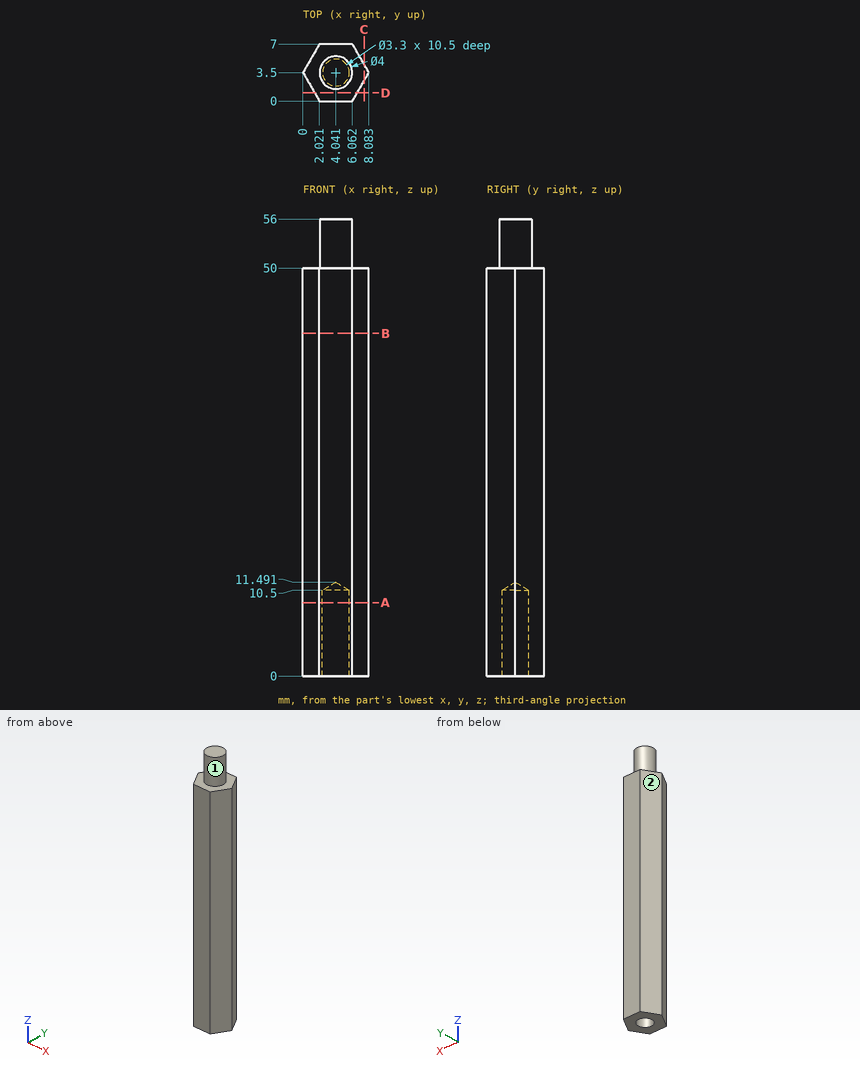
The figure shows three views and two pictorial views of one solid part (mm, origin at its lowest corner). Answer the questions. A direction names the side the tool comes from. Round coordinates to 2 decimals unless told otherwise and drop trailing zeros. Order: outer loops, then holes, each group sorted by start corner. A loop starts at its lowest first (then second) coordinate and runs counter-clockwise, first axis right, second up. Notation, with made-up numbers: M 40.5,35.5 L 84.5,35.5 A18 cw 84.5,45.5 Z; hole C 42,45.25 d7. An arc over 180 degrees is marked long. Put each result on its own line as item: value. Start each with the question number.
Q1. Section D-D, the plane y = 1 is taken. Write down the section's boundary in (x, z).
Q2. Section C-C, the plane x = 7.5 is taken. Write down the section's boundary in (y, z).
Q3. Straight lines are drawn through the part: L1, parallel to X at y = 3.5, z = 6; L2, parallel to Z at x = 6, y = 6.25; L3, parallel to Y at x = 3.5, z = 7.5. For each, find the intervals that lie inside material, in ascending order. Write a range as [from, to].
Q4. Section A-A, the plane z = 9 is taken. Write down the section's boundary in (x, y), and give its area (3 significant figures).
Q5. A tool of negligible diameter and unlimited length cuts with its end or side. For the marked faces 1 and 2, from which of +Z, -Z, +X, -X, +Y, -Y can it reach the whole face along a straight path? Write none if from no direction.
Q6. Flat-ended cylindrical pins translate along their axes: pin 1 (2 mm diameter, centred on y = 2, z = 28, fed in from +X) (1 decimal); pin 2 (3 mm diameter, centred on y = 6, z = 22, fed in from +X) (1 decimal). Find the tip coordinate at first contact, or state that the pin passes through.
Q7. Section B-B, the plane z = 42 is taken. Write down the section's boundary in (x, y).
Findings below:
1. outline: M 1.44,0 L 6.64,0 L 6.64,50 L 1.44,50 Z
2. outline: M 2.49,0 L 4.51,0 L 4.51,50 L 2.49,50 Z
3. L1: x = [0, 2.39], [5.69, 8.08]
3. L2: z = [0, 50]
3. L3: y = [0, 1.94], [5.06, 7]
4. outline: M 0,3.5 L 2.02,0 L 6.06,0 L 8.08,3.5 L 6.06,7 L 2.02,7 Z; hole C 4.04,3.5 d3.3
4. area: 33.9 mm^2
5. face 1: +Z
5. face 2: +Z, -Z, -X, +Y
6. pin 1: stops at x = 7.8
6. pin 2: stops at x = 7.5
7. outline: M 0,3.5 L 2.02,0 L 6.06,0 L 8.08,3.5 L 6.06,7 L 2.02,7 Z
